Study the drawing (mm; zero at the part's minimum x, y, z) and answer. Give positions to 0.01 mm unless a question says otherwise; leave off trailing zeros. Order: outer loops, then holes, each group sorted by start corner. A loop starts at its lowest first (then second) coordinate and runs counter-clockwise, first axis right, second up. Notation, with made-up numbers: (-14, 30.5) - (17, 30.5) arc R19 cw to (17, 53.5) - close; hole circle Ø6 at (64.25, 1.5). An arc over 180 degrees is marked (long way). Put each result on its own line as item: value.
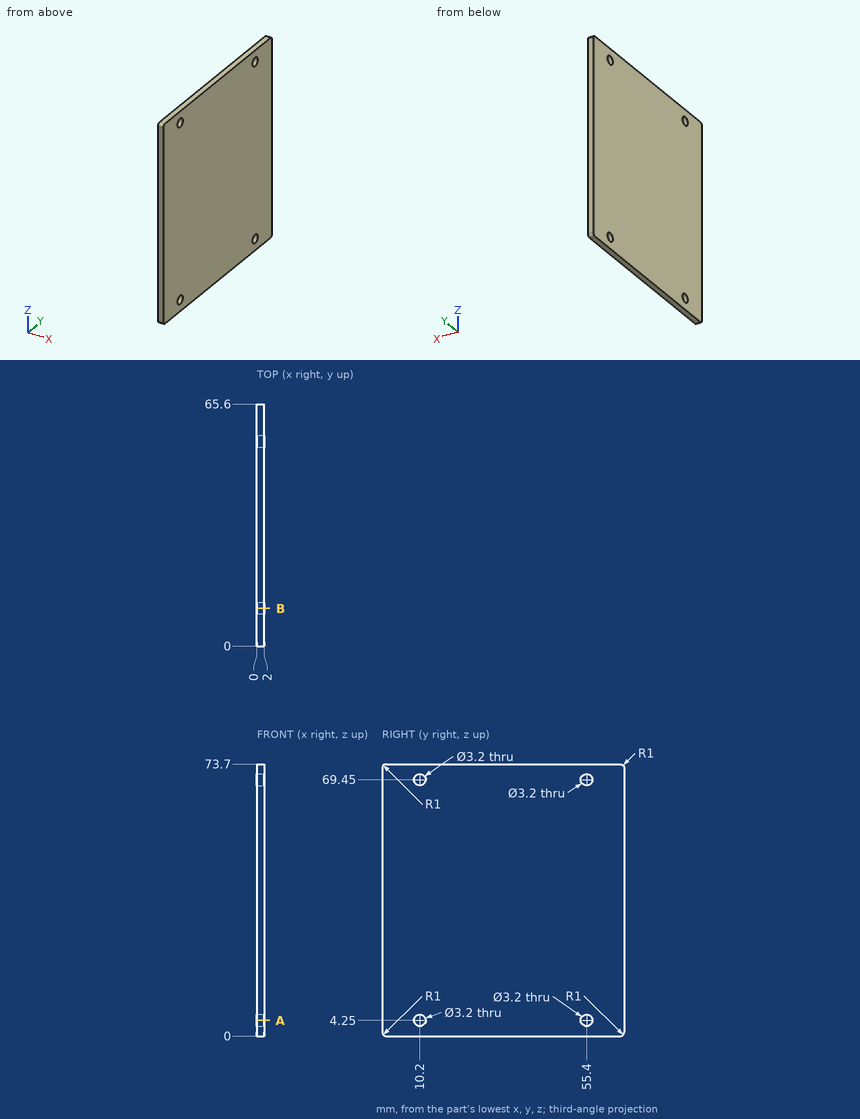
(1) Section A-A, the plane z = 4.25 is taken. Write down the section's boundary in (x, y).
Geometry check:
outline: (0, 0) - (2, 0) - (2, 8.6) - (0, 8.6) - close; (0, 11.8) - (2, 11.8) - (2, 53.8) - (0, 53.8) - close; (0, 57) - (2, 57) - (2, 65.6) - (0, 65.6) - close
(2) Section B-B, the plane y = 10.2 is taken. Write down the section's boundary in (x, z), then the cut area to 3 significant figures.
Geometry check:
outline: (0, 0) - (2, 0) - (2, 2.65) - (0, 2.65) - close; (0, 5.85) - (2, 5.85) - (2, 67.85) - (0, 67.85) - close; (0, 71.05) - (2, 71.05) - (2, 73.7) - (0, 73.7) - close
area: 135 mm²
(3) Straight lines are drawn through the part: line 1 (Y direction, x = 1.5, z = 4.25); line 2 (Z direction, x = 1.7, y = 9); line 3 (Y direction, x = 0.2, z = 5.5). For each, find the intervals that lie inside material, in ascending order.
Geometry check:
line 1: y = 0 to 8.6, 11.8 to 53.8, 57 to 65.6
line 2: z = 0 to 3.19, 5.31 to 68.39, 70.51 to 73.7
line 3: y = 0 to 9.2, 11.2 to 54.4, 56.4 to 65.6
(4) Given pin 1 (3.5 mm diameter, centred on y = 55.4, z = 69.45, fed in from +X); pin 2 (1.9 mm diameter, centred on y = 10.2, z = 69.45, fed in from -X), each flat-ended and moving along its own axis, determine where each tip first touches the part or whether it passes through.
Geometry check:
pin 1: stops at x = 2
pin 2: passes through
